Model file for the job. Use its own axes, mm. A direction names the side the tool comes from. Coordinates: 2 decimals unless noted, no trailing zeros. Loops run counter-clockwise (first coordinate to the right, second up) from the corner with the lowest first, then second, coordinate; pieces in that order, holes last. Notation, with made-up numbers: M 8.5,24 L 49.5,24 A13 cw 49.5,31 Z; hole C 1.25,-18 d8. An arc over 180 degrees is marked long. Write item = value, one per line. Start each with the question number.
from build123d import *

# Parameters (mm, degrees)
SKETCH1_W           = 900
SKETCH1_H           = 230
BOSS_EXTRUDE1_DEPTH = 120
SKETCH2_W           = 3
SKETCH2_H           = 230
CUT_EXTRUDE1_DEPTH  = 3
SKETCH3_W           = 250
SKETCH3_H           = 120
BOSS_EXTRUDE2_DEPTH = 120


with BuildPart() as part:
    # Sketch1 → Boss-Extrude1 (new body)
    with BuildSketch(Plane.XY):
        Rectangle(SKETCH1_W, SKETCH1_H)
    extrude(amount=BOSS_EXTRUDE1_DEPTH)

    # Sketch2 → Cut-Extrude1 (cut)
    with BuildSketch(Plane.XY.offset(120)):
        with Locations((-300, 0)):
            Rectangle(SKETCH2_W, SKETCH2_H)
        with Locations((-150, 0)):
            Rectangle(SKETCH2_W, SKETCH2_H)
        Rectangle(SKETCH2_W, SKETCH2_H)
        with Locations((150, 0)):
            Rectangle(SKETCH2_W, SKETCH2_H)
        with Locations((300, 0)):
            Rectangle(SKETCH2_W, SKETCH2_H)
    extrude(amount=-CUT_EXTRUDE1_DEPTH, mode=Mode.SUBTRACT)

    # Sketch3 → Boss-Extrude2 (add)
    with BuildSketch(Plane.XY.offset(120)):
        with Locations((-150, -5)):
            Rectangle(SKETCH3_W, SKETCH3_H)
    extrude(amount=BOSS_EXTRUDE2_DEPTH)


solid = part.part
Item 1: Pin check, flat tips, straight feed: pin 1 Ø1 at (y, z) = (56.5, 175) entering from +X; pin 2 Ø3 at (x, y) = (-38.5, 65) entering from +Z; pin 3 Ø0.9 at (x, y) = (300, -8.5) entering from +Z; pin 4 Ø8 at (y, z) = (58, 167.5) entering from +X. Stop position of each tip, or through.
Item 2: Cut at D-D (z = 194.5). Give the cut face in (x, y).
Item 3: 3-axis set-ups, long thin cutter, end or side, ignore diameter. For faces 1 (the flat face through (-6, 2, 0)), 2 (the flat face through (-377, 2, 120)), 3 (the flat face through (-152, 55, 179)), 4 (the flat face through (-152, -65, 179)), 5 (the flat face through (-25, -6, 179)): which of +Z, -Z, +X, -X, +Y, -Y reach the whole face in a straight line?
Item 4: Cut at B-B (x = -126). Give the cut face in (y, z), plus the area to 3 significant figures.
Item 5: Cut at C-C (y = 67). Give the cut face in (x, z).
Item 6: Cut at A-A (y = -45). Give the cut face in (x, z), plus the area to 3 significant figures.
Item 7: Probe L1, parallel to Z at x = -323, y = 1; L2, parallel to Y at x = -187, z = 166.5; L3, parallel to X at y = 40.5, z = 173. List the from-to ranges inside material, lowest first.
Reported:
q1.pin_1 = through
q1.pin_2 = 120
q1.pin_3 = 117
q1.pin_4 = -25
q2.outline = M -275,-65 L -25,-65 L -25,55 L -275,55 Z
q3.face_1 = -Z, +X, -X, +Y, -Y
q3.face_2 = +Z, -X, +Y, -Y
q3.face_3 = +Z, +X, -X, +Y
q3.face_4 = +Z, +X, -X, -Y
q3.face_5 = +Z, +X, +Y, -Y
q4.outline = M -115,0 L 115,0 L 115,120 L 55,120 L 55,240 L -65,240 L -65,120 L -115,120 Z
q4.area = 42,000 mm^2
q5.outline = M -450,0 L 450,0 L 450,120 L 301.5,120 L 301.5,117 L 298.5,117 L 298.5,120 L 151.5,120 L 151.5,117 L 148.5,117 L 148.5,120 L 1.5,120 L 1.5,117 L -1.5,117 L -1.5,120 L -148.5,120 L -148.5,117 L -151.5,117 L -151.5,120 L -298.5,120 L -298.5,117 L -301.5,117 L -301.5,120 L -450,120 Z
q6.outline = M -450,0 L 450,0 L 450,120 L 301.5,120 L 301.5,117 L 298.5,117 L 298.5,120 L 151.5,120 L 151.5,117 L 148.5,117 L 148.5,120 L 1.5,120 L 1.5,117 L -1.5,117 L -1.5,120 L -25,120 L -25,240 L -275,240 L -275,120 L -298.5,120 L -298.5,117 L -301.5,117 L -301.5,120 L -450,120 Z; hole M -151.5,117 L -148.5,117 L -148.5,120 L -151.5,120 Z
q6.area = 138,000 mm^2
q7.L1 = 0 to 120
q7.L2 = -65 to 55
q7.L3 = -275 to -25
